Can you work these out from the drawing? Everything is in mm from the part's minimum corner. A direction names the side the tool comes from. Give positions to 0.01 mm unless a question says otherwise; leave off trailing zeros. Write each loop counter-clockwise with the first axis right and the second up, starting at its lowest first coordinate (ties: lowest second). Pieces come first, ordered by that corner, then holes. Notation, with made-up numbers: (37.25, -20) -> (54.25, -20) arc R17 ccw to (54.25, 4) -> close; hole circle Ø2 at (-36.5, 35.25). An arc over 180 degrees is marked (long way). Return JSON: item names as keys, results as strings.
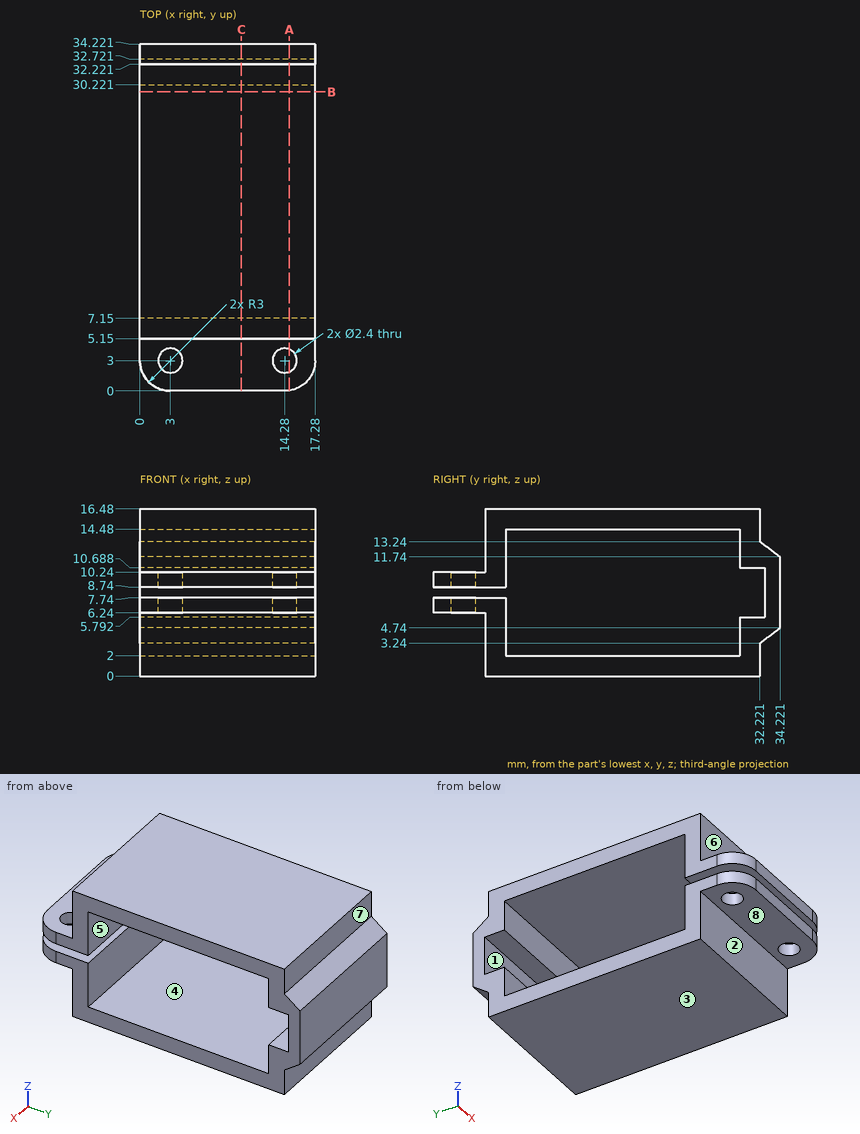
1. If I drill on line 1 (Y direction, x = 3, z = 6.65); line 2 (Z direction, x = 14.75, y = 15); line 3 (Y direction, x = 12.5, z = 9.5), over which ranges is the centre line in solid material (lowest first)? Write a range as [from, to].
Taken from the geometry:
{"line 1": "y = [0, 1.8], [4.2, 7.15], [32.72, 34.22]", "line 2": "z = [0, 2], [14.48, 16.48]", "line 3": "y = [0, 7.15], [32.72, 34.22]"}
2. Suppose I cut it at A-A, the plane x = 14.75. Count the separate pieces of the cut face and the enclosed holes in it, and give its area (3 significant figures).
Taken from the geometry:
{"separate pieces": "3", "enclosed holes": "0", "area": "170 mm²"}
3. Suppose I cut it at C-C, the plane x = 10. List the corners of the cut face in (y, z) for me.
Taken from the geometry:
{"outline": "(0, 6.24) -> (5.15, 6.24) -> (5.15, 0) -> (32.22, 0) -> (32.22, 3.24) -> (34.22, 4.74) -> (34.22, 11.74) -> (32.22, 13.24) -> (32.22, 16.48) -> (5.15, 16.48) -> (5.15, 10.24) -> (0, 10.24) -> (0, 8.74) -> (7.15, 8.74) -> (7.15, 14.48) -> (30.22, 14.48) -> (30.22, 10.69) -> (32.72, 10.69) -> (32.72, 5.79) -> (30.22, 5.79) -> (30.22, 2) -> (7.15, 2) -> (7.15, 7.74) -> (0, 7.74) -> close"}
4. For pin 1 Ø1 at (x, z) = (12, 1) entering from +Y; pin 2 Ø4 at (x, y) = (7, 1.5) entering from +Z; pin 3 Ø1.5 at (x, z) = (14, 13) entering from -Y, each with a flat end and sliding along its axis, tell me the tip position at first contact or that it passes through.
Taken from the geometry:
{"pin 1": "stops at y = 32.22", "pin 2": "stops at z = 10.24", "pin 3": "stops at y = 5.15"}
5. If we mould it in two halves opening along Y, with no side actions, what happens to the marked faces 1, 2, 3 and 4? For each: released by +Y, released by -Y, zero draft, split by the parting line, or undercut.
Taken from the geometry:
{"face 1": "undercut", "face 2": "released by -Y", "face 3": "zero draft", "face 4": "undercut"}
6. Suppose I cut it at B-B, the plane y = 29.5. List the corners of the cut face in (x, z) for me.
Taken from the geometry:
{"outline": "(0, 0) -> (17.28, 0) -> (17.28, 2) -> (0, 2) -> close; (0, 14.48) -> (17.28, 14.48) -> (17.28, 16.48) -> (0, 16.48) -> close"}
7. Which directions (+Z, -Z, +X, -X, +Y, -Y) give clear straight access to the entire face, cutting with the end or side of a thin tool? Please do the marked faces 5, 6, 7 and 8.
Taken from the geometry:
{"face 5": "+X, -X", "face 6": "+Z, +X, -X, -Y", "face 7": "+Z, +X, -X, +Y", "face 8": "-Z, +X, -X, -Y"}
